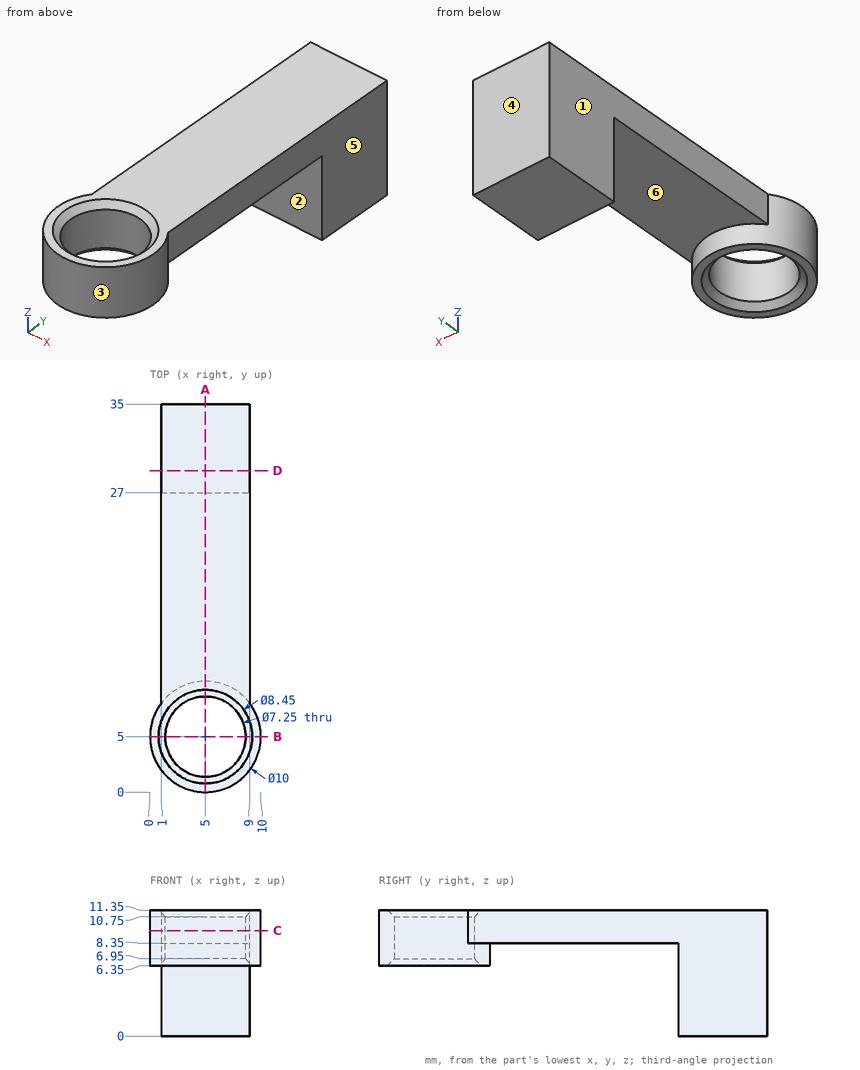
Check sheet for the drawn part. Datum: minimum x, y, z corner. Units: mm. A direction names the side the tool comes from. Give positions to 0.01 mm unless a question says otherwise; leave off trailing zeros. Loops run counter-clockwise (first coordinate to the right, second up) from the corner with the lowest first, then second, coordinate; pieces in that order, holes last.
1) Set-up check for the marked faces 1, 2 and 3: record each of +Z, -Z, +X, -X, +Y, -Y from which the full face is reachable in a straight line by a thin tool's end or side.
2) Thickness scan on line 1 along Y through (x, z) = (5, 8) (3 decimals); line 2 along Y through (x, z) = (2, 7.5); line 3 along Y through (x, z) = (5, 8.6) (3 decimals). Record the ranges inside material, lowest first.
3) Depth check by flat-ended pin: pin 1 Ø1.5 at (y, z) = (22, 9.5) entering from +X; pin 2 Ø2 at (x, y) = (8.5, 14) entering from -Z; pin 3 Ø6 at (y, z) = (30.5, 4) entering from -X. Enter the tip coordinate at first touch or a pass-through.
4) Sectioned sample at A-A, the plane x = 5. Enter the section's corners in (y, z) (3 decimals).
5) Sectioned sample at D-D, the plane y = 29. Enter the section's corners in (x, z).
6) Sectioned sample at C-C, the plane z = 9.5. Enter the section's corners in (x, y) (3 decimals).
7) Draft check along Y on the marked faces 4, 5 and 6. Enter one of: pulls with the +Y half, pulls with the -Y half, needs draft (parallel to the pull), parting line crosses it, or undercut.
8) Sectioned sample at B-B, the plane y = 5. Enter the section's corners in (x, z) (3 decimals).
Answers:
1. face 1: +Z, -Z, -X, +Y
1. face 2: -Z, +X, -X
1. face 3: -Z
2. line 1: y = 0 to 1.375, 8.625 to 10, 27 to 35
2. line 2: y = 1 to 2.97, 7.03 to 9, 27 to 35
2. line 3: y = 0 to 1.375, 8.625 to 35
3. pin 1: stops at x = 9
3. pin 2: stops at z = 8.35
3. pin 3: stops at x = 1
4. outline: (0, 6.35) - (0.775, 6.35) - (1.375, 6.95) - (1.375, 10.75) - (0.775, 11.35) - (0, 11.35) - close; (8.625, 6.95) - (9.225, 6.35) - (10, 6.35) - (10, 8.35) - (27, 8.35) - (27, 0) - (35, 0) - (35, 11.35) - (9.225, 11.35) - (8.625, 10.75) - close
5. outline: (1, 0) - (9, 0) - (9, 11.35) - (1, 11.35) - close
6. outline: (1, 8) arc R5 ccw (long way) to (9, 8) - (9, 35) - (1, 35) - close; hole circle Ø7.25 at (5, 5)
7. face 4: pulls with the +Y half
7. face 5: needs draft
7. face 6: undercut
8. outline: (0, 6.35) - (0.775, 6.35) - (1.375, 6.95) - (1.375, 10.75) - (0.775, 11.35) - (0, 11.35) - close; (8.625, 6.95) - (9.225, 6.35) - (10, 6.35) - (10, 11.35) - (9.225, 11.35) - (8.625, 10.75) - close
